from build123d import *

# Parameters (mm, degrees)
F1_DEPTH = 38.1
F3_DEPTH = 25.4


with BuildPart() as f1:
    # F0 (on Right) → F1 (new body)
    with BuildSketch(Plane.YZ):
        Polygon((0, 25.4), (0, 0), (25.4, 0), (25.4, 25.4), (19.05, 25.4), (19.05, 12.7), (6.35, 12.7), (6.35, 25.4), align=None)
    extrude(amount=F1_DEPTH)

    # F2 (on Front) → F3 (cut)
    with BuildSketch(Plane.XZ):
        Polygon((38.1, 25.4), (19.05, 25.4), (38.1, 0), align=None)
    extrude(amount=-F3_DEPTH, mode=Mode.SUBTRACT)


solid = f1.part
The model under review builds one solid part; all positions refer to its coordinate system, in mm. A direction names the side the tool comes from. Round coordinates to 2 decimals unless told otherwise and drop trailing zeros. Loops run counter-clockwise (first coordinate to the right, second up) from the corner with the lowest first, then second, coordinate; pieces in that order, holes last. Notation, with made-up numbers: M -37,86.5 L -19,86.5 A13 ccw -19,111.5 Z; hole C 50,75.25 d1. An arc over 180 degrees is marked long. Answer as a JSON object with one key per item and string values.
Item 1: Tool access review of faces 1 (the face through (30.558, 12.522, 10.056)), 2 (the face through (11, 6.35, 19)): name each direction out of +Z, -Z, +X, -X, +Y, -Y from which nothing blocks a thin tool from reaching the whole face with its end or side.
Check sheet entries:
{"face 1": "+Z, +X, +Y, -Y", "face 2": "+Z, +X, -X"}
Item 2: We need section B-B, the plane x = 7. State the section outline as (y, z) points, and give its area (3 significant figures).
Check sheet entries:
{"outline": "M 0,0 L 25.4,0 L 25.4,25.4 L 19.05,25.4 L 19.05,12.7 L 6.35,12.7 L 6.35,25.4 L 0,25.4 Z", "area": "484 mm2"}
Item 3: We need section D-D, the plane y = 15.25. State the section outline as (x, z) points (3 decimals).
Check sheet entries:
{"outline": "M 0,0 L 38.1,0 L 28.575,12.7 L 0,12.7 Z"}
Item 4: We need section A-A, the plane z = 21. State the section outline as (x, y) points, and give its area (3 significant figures).
Check sheet entries:
{"outline": "M 0,0 L 22.35,0 L 22.35,6.35 L 0,6.35 Z; M 0,19.05 L 22.35,19.05 L 22.35,25.4 L 0,25.4 Z", "area": "284 mm2"}
Item 5: For line 1 along Y through (x, z) = (6.5, 16.75); line 2 along Z through (x, y) = (15, 17.75); line 3 along X through (y, z) = (5.25, 5.75), list the stretches that pass through material, from the lowest coordinate up.
Check sheet entries:
{"line 1": "0 to 6.35, 19.05 to 25.4", "line 2": "0 to 12.7", "line 3": "0 to 33.79"}
Item 6: Clearance check with flat-ended pins moving along their axes: P1, Ø10, axis at y = 2.5, z = 10.5, coming from the +X side (3 decimals); P2, Ø10, axis at x = 16.5, y = 12, coming from the +Z side. State where each tip first meets the part, or that it passes through.
Check sheet entries:
{"P1": "x = 33.975", "P2": "z = 12.7"}
Item 7: We need section C-C, the plane z = 16. State the section outline as (x, y) points, and give its area (3 significant figures).
Check sheet entries:
{"outline": "M 0,0 L 26.1,0 L 26.1,6.35 L 0,6.35 Z; M 0,19.05 L 26.1,19.05 L 26.1,25.4 L 0,25.4 Z", "area": "331 mm2"}
Item 8: The part is to be moulded in two halves that separate along Y. For faces 3 (the face through (9, 22, 25.4)), 4 (the face through (14, 13, 12.7)), 5 (the face through (11, 19.05, 19)), 6 (the face through (15, 0, 13)), say which applies: +Y half, -Y half, draft (parallel to the pull), parting line (faces both ways), or undercut.
Check sheet entries:
{"face 3": "draft", "face 4": "undercut", "face 5": "undercut", "face 6": "-Y half"}
